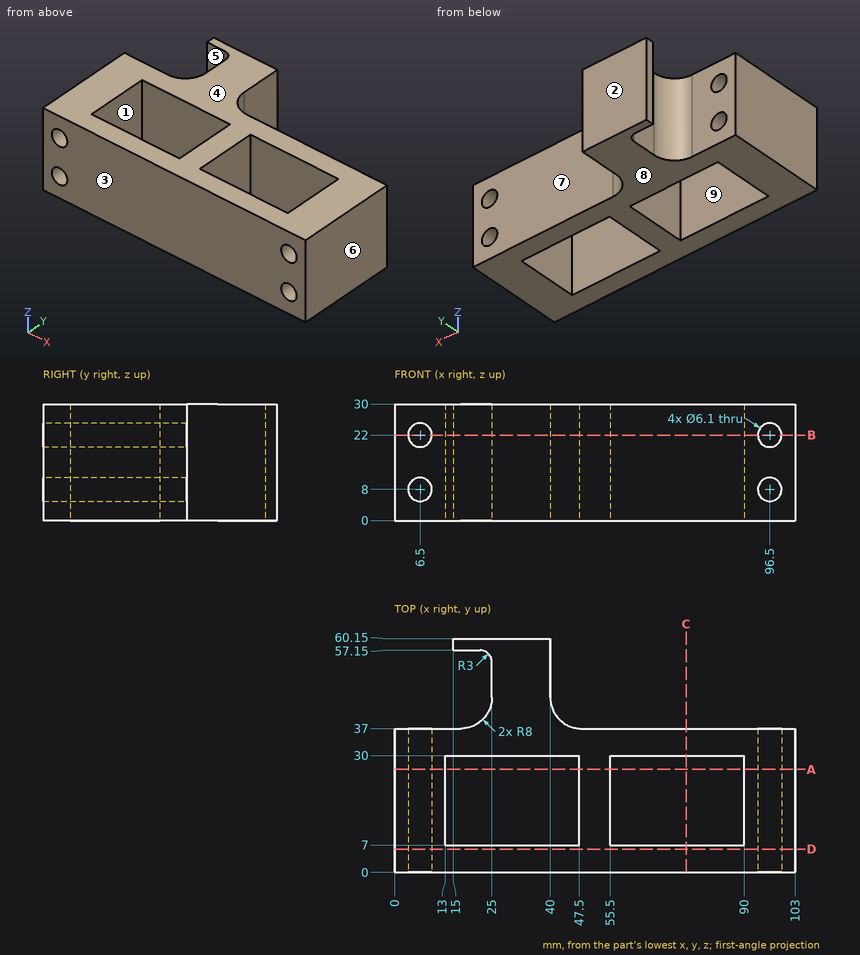
Design review of the part shown in the three views and the two pictorial views. Dimensions are in mm from the part's minimum x, y and z. A direction names the side the tool comes from. Round coordinates to 2 decimals unless told otherwise and drop trailing zeros. Loops run counter-clockwise (first coordinate to the right, second up) from the corner with the lowest first, then second, coordinate; pieces in that order, holes last. Notation, with made-up numbers: (41.25, -25) -> (60.25, -25) arc R14 ccw to (60.25, -7) -> close; hole circle Ø11 at (3.5, 21.25). An arc over 180 degrees is marked (long way). Return JSON: item names as keys, results as strings.
(1) Add section A-A on y = 26.5. Write out the cut boundary in (x, z).
Solved:
{"outline": "(0, 0) -> (13, 0) -> (13, 30) -> (0, 30) -> close; (47.5, 0) -> (55.5, 0) -> (55.5, 30) -> (47.5, 30) -> close; (90, 0) -> (103, 0) -> (103, 30) -> (90, 30) -> close; hole circle Ø6.1 at (6.5, 8); hole circle Ø6.1 at (6.5, 22); hole circle Ø6.1 at (96.5, 8); hole circle Ø6.1 at (96.5, 22)"}
(2) Add section D-D on y = 6. Write out the cut boundary in (x, z).
Solved:
{"outline": "(0, 0) -> (103, 0) -> (103, 30) -> (0, 30) -> close; hole circle Ø6.1 at (6.5, 8); hole circle Ø6.1 at (6.5, 22); hole circle Ø6.1 at (96.5, 8); hole circle Ø6.1 at (96.5, 22)"}
(3) For the marked faces 5, 6, 7, 8 and 9, list the 3-axis set-ups (+Z, -Z, +X, -X, +Y, -Y) from which the entire face can be reached by the end or side of a thin tool; tool diameter is ignored.
Solved:
{"face 5": "+Z, -Z, -X", "face 6": "+Z, -Z, +X, +Y, -Y", "face 7": "+Z, -Z, +X, +Y", "face 8": "-Z, +X, -X, +Y, -Y", "face 9": "+Z, -Z"}
(4) For line 1 (X direction, y = 12.5, z = 8); line 2 (X direction, y = 12, z = 28.5); line 3 (X direction, y = 4.5, z = 22.25), list the stretches that pass through material, from the lowest coordinate up.
Solved:
{"line 1": "0 to 3.45, 9.55 to 13, 47.5 to 55.5, 90 to 93.45, 99.55 to 103", "line 2": "0 to 13, 47.5 to 55.5, 90 to 103", "line 3": "0 to 3.46, 9.54 to 93.46, 99.54 to 103"}
(5) Add section C-C on x = 75. Write out the cut boundary in (y, z).
Solved:
{"outline": "(0, 0) -> (7, 0) -> (7, 30) -> (0, 30) -> close; (30, 0) -> (37, 0) -> (37, 30) -> (30, 30) -> close"}
(6) The part is to be moulded in two halves that separate along Y. For the marked faces 1, 2, 3 and 4, say which applies: released by +Y, released by -Y, zero draft, split by the parting line, or undercut.
Solved:
{"face 1": "undercut", "face 2": "released by +Y", "face 3": "released by -Y", "face 4": "zero draft"}
(7) Add section B-B on z = 22. State how many separate pieces and enclosed holes the cut face has, plus the area to 3 significant figures.
Solved:
{"separate pieces": "3", "enclosed holes": "2", "area": "2,180 mm2"}
(8) For pin 1 (5 mm diameter, centred on x = 26, y = 29, fed in from -Z); pin 2 (12 mm diameter, centred on y = 53, z = 18, fed in from +X); pin 3 (15 mm diameter, centred on x = 78.5, z = 10, fed in from +Y); pin 4 (12 mm diameter, centred on y = 48.5, z = 10.5, fed in from +X), all flat-tipped, find the tip position at first contact; note any pin that passes through.
Solved:
{"pin 1": "z = 0", "pin 2": "x = 40", "pin 3": "y = 37", "pin 4": "x = 40.4"}
